Read the model definition and answer for the solid it produces. Units are mm, in the model's axes. A direction names the side the tool comes from. Give positions to 0.01 mm unless a question says otherwise; leave off trailing zeros. Order: outer loops, then holes, each group sorted by start corner. A loop starts at its lowest first (then second) coordinate and runs counter-clockwise, first axis right, second up. Notation, with made-up numbers: (43, -25) -> (79, -25) arc R28 cw to (79, -4) -> close; hole circle Ø8 at (32, 65). An arc over 180 degrees is marked (long way). One line per item, written item: value. Start each with the question number.
from build123d import *

# Parameters (mm, degrees)
SKETCH1_R           = 53.848
EXTRUDE1_DEPTH      = 127.7874
SKETCH13_W          = 15.1892
SKETCH13_H          = 36.2585
S2D0011_W           = 8.7376
S2D0011_H           = 18.034
SKETCH16_W          = 123.825
SKETCH16_H          = 50.546
EXTRUDE2_DEPTH      = 60.325
SKETCH17_R          = 10.4775
CUT_EXTRUDE9_DEPTH  = 0.254
SKETCH18_R          = 10.4775
CUT_EXTRUDE10_DEPTH = 0.254
SKETCH21_R          = 6.9469
EXTRUDE3_DEPTH      = 1.27
CHAMFER1_SIZE       = 1.1684
CHAMFER1_SIZE2      = 0.674576055


with BuildPart() as part:
    # Sketch1 → Extrude1 (new body)
    with BuildSketch(Plane.XY):
        Circle(SKETCH1_R)
    extrude(amount=EXTRUDE1_DEPTH)

    # Sketch10 → Cut-Revolve1 (revolve, cut)
    with BuildSketch(Plane(origin=(0, 0, 0), x_dir=(0, 0, -1), z_dir=(1, 0, 0)), mode=Mode.PRIVATE) as cut_revolve1_sk:
        Polygon((-127.7874, 52.8447), (-107.5436, 52.8447), (-106.5403, 53.848), (-127.7874, 53.848), align=None)
    revolve(cut_revolve1_sk.sketch.rotate(Axis((0, 0, 160.082178917), (0, 0, -1)), 90), axis=Axis((0, 0, 160.082178917), (0, 0, -1)), mode=Mode.SUBTRACT)  # turned: the seam where the file's is

    # Sketch13 → Revolve1 (revolve)
    with BuildSketch(Plane(origin=(0, 0, 0), x_dir=(0, 0, -1), z_dir=(1, 0, 0)), mode=Mode.PRIVATE) as revolve1_sk:
        with Locations((-135.382, 18.12925)):
            Rectangle(SKETCH13_W, SKETCH13_H)
    revolve(revolve1_sk.sketch.rotate(Axis((0, 0, 113.59896), (0, 0, -1)), 90), axis=Axis((0, 0, 113.59896), (0, 0, -1)))  # turned: the seam where the file's is

    # S2D0011 → Cut-Revolve4 (revolve, cut)
    with BuildSketch(Plane(origin=(-6.9342, 0, 112.8014), x_dir=(-1, 0, 0), z_dir=(0, 1, 0)), mode=Mode.PRIVATE) as cut_revolve4_sk:
        with Locations((-2.5654, 21.1582)):
            Rectangle(S2D0011_W, S2D0011_H)
    revolve(cut_revolve4_sk.sketch.rotate(Axis((0, 0, 106.5403), (0, 0, 1)), 180), axis=Axis((0, 0, 106.5403), (0, 0, 1)), mode=Mode.SUBTRACT)  # turned: the seam where the file's is

    # Sketch15 → Cut-Revolve5 (revolve, cut)
    with BuildSketch(Plane(origin=(0, 0, 0), x_dir=(0, 0, -1), z_dir=(1, 0, 0)), mode=Mode.PRIVATE) as cut_revolve5_sk:
        with BuildLine():
            Line((-142.9766, 26.9875), (-140.585166919, 35.66172482))
            ThreePointArc((-140.585166919, 35.66172482), (-140.294072774, 36.092317667), (-139.8016, 36.2585))
            Line((-139.8016, 36.2585), (-142.9766, 36.2585))
            Line((-142.9766, 36.2585), (-142.9766, 26.9875))
        make_face()
    revolve(cut_revolve5_sk.sketch.rotate(Axis((0, 0, 112.96015), (0, 0, -1)), 90), axis=Axis((0, 0, 112.96015), (0, 0, -1)), mode=Mode.SUBTRACT)  # turned: the seam where the file's is

    # Sketch16 → Extrude2 (add, symmetric)
    with BuildSketch(Plane(origin=(0, 0, 0), x_dir=(-1, 0, 0), z_dir=(0, 1, 0))):
        with Locations((-1.5875, -1.7272)):
            Rectangle(SKETCH16_W, SKETCH16_H)
    extrude(amount=EXTRUDE2_DEPTH, both=True)

    # Sketch17 → Cut-Extrude9 (cut)
    with BuildSketch(Plane(origin=(63.5, 0, 0), x_dir=(0, 0, -1), z_dir=(1, 0, 0))):
        with Locations((17.7292, -31.75)):
            Circle(SKETCH17_R)
    extrude(amount=-CUT_EXTRUDE9_DEPTH, mode=Mode.SUBTRACT)

    # Sketch18 → Cut-Extrude10 (cut)
    with BuildSketch(Plane(origin=(63.5, 0, 0), x_dir=(0, 0, -1), z_dir=(1, 0, 0))):
        with Locations((17.7292, 31.75)):
            Circle(SKETCH18_R)
    extrude(amount=-CUT_EXTRUDE10_DEPTH, mode=Mode.SUBTRACT)

    # S2D0001 → Cut-Revolve7 (revolve, cut)
    with BuildSketch(Plane(origin=(52.1462, 23.8125, -17.7292), x_dir=(0, -1, 0), z_dir=(0, 0, 1)), mode=Mode.PRIVATE) as cut_revolve7_sk:
        Polygon((-7.9375, 11.0998), (-1.7526, 11.0998), (-2.295193135, 8.5471), (-2.9591, 7.883193135), (-2.9591, -6.1722), (-7.9375, -6.1722), align=None)
    revolve(cut_revolve7_sk.sketch.rotate(Axis((34.0106, 31.75, -17.7292), (1, 0, 0)), 270), axis=Axis((34.0106, 31.75, -17.7292), (1, 0, 0)), mode=Mode.SUBTRACT)  # turned: the seam where the file's is

    # Sketch21 → Extrude3 (add)
    with BuildSketch(Plane(origin=(63.246, 0, 0), x_dir=(0, 0, -1), z_dir=(1, 0, 0))):
        with Locations((17.7292, -31.75)):
            Circle(SKETCH21_R)
    extrude(amount=EXTRUDE3_DEPTH)

    # Chamfer1
    chamfer1_edges = [part.edges().sort_by_distance(p)[0] for p in [
        (-8.7376, 0, 142.9766),
    ]]
    chamfer1_side = [part.faces().sort_by_distance(p)[0] for p in [
        (-8.7376, 0, 133.9596),
    ]]
    chamfer(chamfer1_edges, length=CHAMFER1_SIZE, length2=CHAMFER1_SIZE2, reference=chamfer1_side[0])

    # Sketch23 → Cut-Revolve8 (revolve, cut)
    with BuildSketch(Plane(origin=(0, 0, 0), x_dir=(0, 0, -1), z_dir=(1, 0, 0))):
        Polygon((-121.5517, 52.8447), (-121.5517, 44.9707), (-116.6622, 42.032792003), (-116.6622, 52.8447), align=None)
    cut_revolve8 = revolve(axis=Axis((0, 62.163785144, 116.6622), (0, -1, 0)), mode=Mode.SUBTRACT)

    # Mirror1: Cut-Revolve8 across plane
    add(cut_revolve8.mirror(Plane.ZX), mode=Mode.SUBTRACT)


solid = part.part
Item 1: Find section A-A on y = 0. Write down the section's boundary in (x, z) (1 decimal), then the cut area to 3 significant figures.
Item 2: Flat-ended cylindrical pins translate along their axes: pin 1 (2 mm diameter, centred on y = 16, z = 23, fed in from +X); pin 2 (4 mm diameter, centred on x = 20, y = 26.5, fed in from +Z); pin 3 (11 mm diameter, centred on x = 0, z = 116.66, fed in from -Y). Find the tip coordinate at first contact, or state that the pin passes through.
Item 3: A tool of negligible diameter and unlimited length cuts with its end or side. For faces 4 (the flat face through (-12.5, -34.5, 127.787)), 5 (the flat face through (2, 60.325, -1)), 6 (the cylindrical face through (-1.469, 48.853, 121.326)), 7 (the cylindrical face through (63.87, -38.53, -16.22)), from which of +Z, -Z, +X, -X, +Y, -Y can it reach the whole face along a straight path? Write none if from no direction.
Item 4: Find section B-B on z = 32.5. Write down the section's boundary in (x, y), then the cut area to 3 significant figures.
Item 5: For a pull along Z with two mould halves and no side action, classify faces 1 (the cylindrical face through (52.9, 36.61, -18.81)), 2 (the cylindrical face through (-36.223, -1.594, 133.71)), 3 (the conical face through (-5.968, 26.875, 142.827)) as +Z half, -Z half, draft (parallel to the pull), parting line (faces both ways), or undercut.
Item 6: Find the intervals of material crossed by line 1 (Z direction, x = 0, y = -48.75); line 2 (Y direction, x = 0, z = 129); line 3 (X direction, y = -10.5, z = 50.5), in increasing order. Write a range as from..to.
Checks:
1. outline: (-60.3, -27) -> (63.5, -27) -> (63.5, 23.5) -> (53.8, 23.5) -> (53.8, 106.5) -> (52.8, 107.5) -> (52.8, 127.8) -> (36.3, 127.8) -> (36.3, 139.8) arc R0.8 ccw to (35.7, 140.6) -> (27, 143) -> (9.4, 143) -> (8.7, 141.8) -> (8.7, 124.9) -> (-8.7, 124.9) -> (-8.7, 141.8) -> (-9.4, 143) -> (-27, 143) -> (-35.7, 140.6) arc R0.8 ccw to (-36.3, 139.8) -> (-36.3, 127.8) -> (-52.8, 127.8) -> (-52.8, 107.5) -> (-53.8, 106.5) -> (-53.8, 23.5) -> (-60.3, 23.5) -> close
1. area: 18,200 mm2
2. pin 1: x = 63.5
2. pin 2: z = 141.82
2. pin 3: y = -52.84
3. face 4: +Z
3. face 5: +Z, -Z, +X, -X, +Y
3. face 6: +Y
3. face 7: +X
4. outline: circle Ø107.7 at (0, 0)
4. area: 9,110 mm2
5. face 1: undercut
5. face 2: draft
5. face 3: +Z half
6. line 1: -27..111.77, 121.55..127.79
6. line 2: -36.26..-8.74, 8.74..36.26
6. line 3: -52.81..52.81
